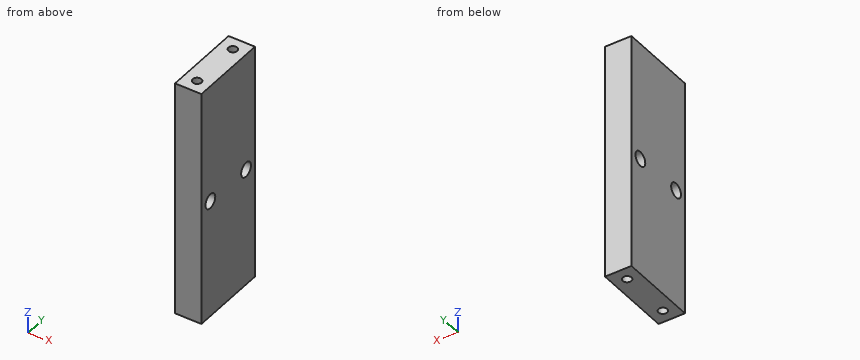
Autodesk Inventor part; units mm, degrees
ref_plane "YZ Plane" through (0, 0, 0) normal (1, 0, 0) x (0, 1, 0)
ref_plane "XZ Plane" through (0, 0, 0) normal (0, 1, 0) x (-1, 0, 0)
ref_plane "XY Plane" through (0, 0, 0) normal (0, 0, 1) x (1, 0, 0)
sketch "スケッチ1" plane through (0, 0, 0) normal (0, 0, 1) x (1, 0, 0)
  line L0 (-5, -15) -> (5, -15)
  line L1 (5, -15) -> (5, 15)
  line L2 (5, 15) -> (-5, 15)
  line L3 (-5, 15) -> (-5, -15)
  line L4 (-5, -15) -> (5, 15) construction
  line L5 (5, -15) -> (-5, 15) construction
  point P0 (0, 0)
  dimension "d0" = 10
  dimension "d1" = 30
extrude "押し出し1" add sketch "スケッチ1" along normal mid plane 90
sketch "スケッチ2" plane through (0, 0, 45) normal (0, 0, 1) x (1, 0, 0)
  line L0 (5, 15) -> (-5, 15)
  line L1 (5, -15) -> (5, 15)
  line L2 (-5, -15) -> (5, -15)
  point P0 (0, 0)
  point P1 (0, 10)
  point P2 (0, -10)
  dimension "d4" = 5
  dimension "d5" = 5
  dimension "d6" = 5
  dimension "d7" = 5
hole "穴1" at (0, 10, 45) at (0, -10, 45) direction (0, 0, -1) diameter 3.3 depth 10 tip angle 118
sketch "スケッチ3" plane through (0, 0, -45) normal (0, 0, -1) x (-1, 0, 0)
  circle A0 centre (0, 10) radius 1.65
  circle A1 centre (0, -10) radius 1.65
  point P0 (0, 0)
hole "穴2" at (0, 10, -45) at (0, -10, -45) direction (0, 0, 1) diameter 3.3 depth 10 tip angle 118
sketch "スケッチ4" plane through (5, -15, 45) normal (1, 0, 0) x (0, 0, -1)
  line L0 (90, 30) -> (0, 30)
  line L1 (0, 0) -> (0, 30)
  point P0 (45, 15)
  point P1 (45, 25)
  point P2 (45, 5)
  point P3 (45, 30)
  dimension "d22" = 5
  dimension "d23" = 20
  dimension "d24" = 45
  dimension "d25" = 45
hole "穴3" at (5, 10, 0) at (5, -10, 0) direction (-1, 0, 0) diameter 5.5 end through all
properties part number "base_part_attachment_ver2"
Check sheet for the modelled part. Datum: model origin and axes. Units: mm. Round coordinates to 2 decimals unless told otherwise and drop trailing zeros. Loops run counter-clockwise (first coordinate to the right, second up) from the corner with the lowest first, then second, coordinate; pieces in that order, holes last. Notation, with made-up numbers: M 65.5,-5 L 117.5,-5 A21 ccw 117.5,31 Z; hole C 76.25,-30 d11. An arc over 180 degrees is marked long. One line per item, written item: value.
(1) Sectioned sample at C-C, the plane z = 39.5. Record the cut outline in (x, y).
Computed values:
outline: M -5,-15 L 5,-15 L 5,15 L -5,15 Z; hole C 0,-10 d3.3; hole C 0,10 d3.3
(2) Thickness scan on line 1 (Y direction, x = 0, z = 43.25); line 2 (Y direction, x = 2.75, z = 0); line 3 (X direction, y = 10, z = -38.5). Record the ranges inside material, lowest first.
Computed values:
line 1: y = -15 to -11.65, -8.35 to 8.35, 11.65 to 15
line 2: y = -15 to -12.75, -7.25 to 7.25, 12.75 to 15
line 3: x = -5 to -1.65, 1.65 to 5
(3) Sectioned sample at B-B, the plane z = 0. Record the cut outline in (x, y), then the cut area to 3 significant figures.
Computed values:
outline: M -5,-15 L 5,-15 L 5,-12.75 L -5,-12.75 Z; M -5,-7.25 L 5,-7.25 L 5,7.25 L -5,7.25 Z; M -5,12.75 L 5,12.75 L 5,15 L -5,15 Z
area: 190 mm^2
(4) Sectioned sample at A-A, the plane x = 3. Record the cut outline in (y, z).
Computed values:
outline: M -15,-45 L 15,-45 L 15,45 L -15,45 Z; hole C -10,0 d5.5; hole C 10,0 d5.5
(5) Depth check by flat-ended pin: pin 1 Ø2 at (x, y) = (0, 10) entering from -Z; pin 2 Ø3 at (x, y) = (-1.5, -9.5) entering from -Z; pin 3 Ø3 at (x, y) = (0, -10) entering from -Z; pin 4 Ø4.5 at (y, z) = (-10, 0) entering from +X. Enter the tip coordinate at first touch or a pass-through.
Computed values:
pin 1: stops at z = -34.61
pin 2: stops at z = -45
pin 3: stops at z = -34.91
pin 4: passes through
